Can you work these out from the drawing? Everything is in mm from the part's minimum corner. A direction names the side the tool comes from. Coordinates: 2 decimals unless noted, no trailing zeros. Order: outer loops, then holes, each group sorted by start corner. A loop starts at its lowest first (then second) coordinate and runs counter-clockwise, first axis right, second up. Notation, with made-up numbers: (26.25, 38.5) -> (62.25, 38.5) arc R20 cw to (62.25, 58.5) -> close; hole circle Ø6 at (15.5, 81). An arc over 180 degrees is marked (long way). Use a Markdown table: item, result. Add a question column.
1) Will these pins go through, and if not, where does the flat tip stop? pin 1 Ø23 at (x, y) = (33, 19.5) entering from +Z; pin 2 Ø1.5 at (x, z) = (22.5, 1) entering from -Y; pin 3 Ø1.5 at (y, z) = (39.5, 4) entering from -X.
2) Which directions (+Z, -Z, +X, -X, +Y, -Y) give clear straight access to the entire face, cutting with the end or side of a thin tool? Please do the marked faces 4 and 5.
3) If I drill on L1, parallel to Y at x = 30, z = 4.15; L2, parallel to Z at x = 36, y = 47; L3, parallel to X at y = 49, z = 4, over which ranges is the centre line in solid material (lowest first)? Write a range as [from, to].
4) If we section it at A-A (x = 30): Write out the boundary of the cut face in (y, z), plus the area to 3 significant figures.
5) If we section it at C-C (z = 5.5): Write out the boundary of the cut face in (x, y).
6) If we section it at D-D (z = 0.75): Write out the boundary of the cut face in (x, y).
7) Thinking about a two-plate mould opening in Y: for the marked faces 1, 2 and 3, which applies, +Y half, -Y half, draft (parallel to the pull), parting line (faces both ways), or undercut?
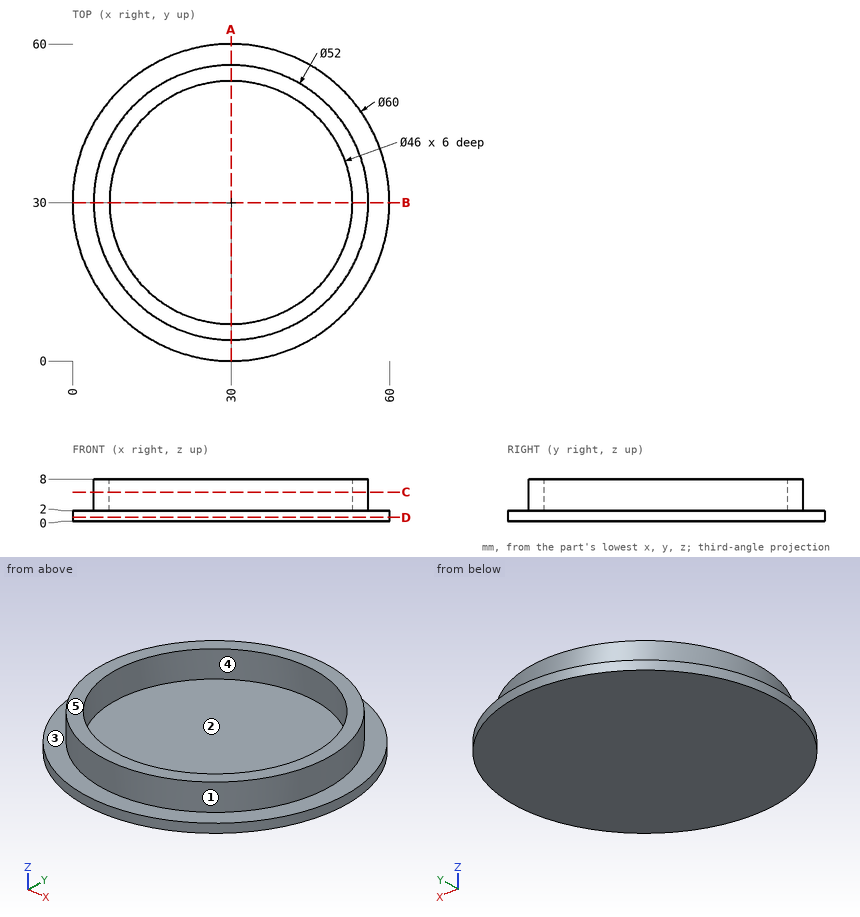
Answer sheet:
| question | item | result |
|---|---|---|
| 1 | pin 1 | z = 2 |
| 1 | pin 2 | y = 0.77 |
| 1 | pin 3 | x = 5.52 |
| 2 | face 4 | +Z |
| 2 | face 5 | +Z, +X, -X, +Y, -Y |
| 3 | L1 | [4, 7], [53, 56] |
| 3 | L2 | [0, 2] |
| 3 | L3 | [12.25, 17.04], [42.96, 47.75] |
| 4 | outline | (0, 0) -> (60, 0) -> (60, 2) -> (56, 2) -> (56, 8) -> (53, 8) -> (53, 2) -> (7, 2) -> (7, 8) -> (4, 8) -> (4, 2) -> (0, 2) -> close |
| 4 | area | 156 mm2 |
| 5 | outline | circle Ø52 at (30, 30); hole circle Ø46 at (30, 30) |
| 6 | outline | circle Ø60 at (30, 30) |
| 7 | face 1 | parting line |
| 7 | face 2 | undercut |
| 7 | face 3 | draft |
